Here's how the part is built. I have some questions about the finished solid (model axes, mm). Face numbers are marked on the shaded views. A direction names the side the tool comes from. Round coordinates to 2 decimals unless told otherwise and drop trailing zeros. Write each loop counter-clockwise with the first axis right and the second up, starting at its lowest first coordinate (ties: lowest second). Pieces come first, ordered by that corner, then holes. Notation, with made-up numbers: (7.5, 85.25) -> (34.5, 85.25) arc R8 ccw to (34.5, 94.25) -> close; hole circle Ø10 at (71.25, -36). An arc over 180 degrees is marked (long way). Answer in a Markdown table with one row per item.
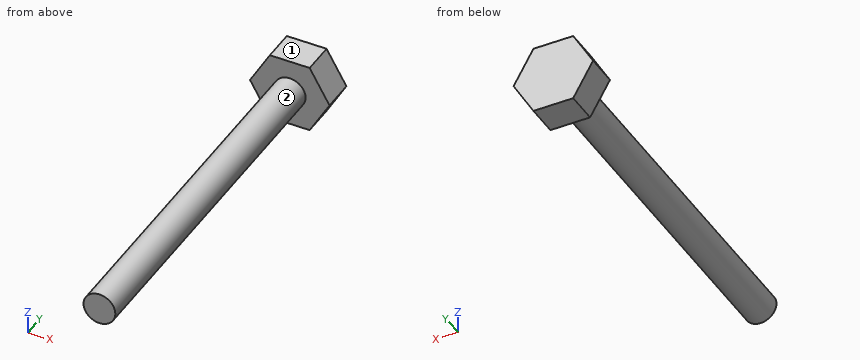
from build123d import *

# Parameters (mm, degrees)
SALIENTE_EXTRUIR1_DEPTH = 4
CROQUIS2_R              = 2
SALIENTE_EXTRUIR2_DEPTH = 45


with BuildPart() as part:
    # Croquis1 → Saliente-Extruir1 (new body)
    with BuildSketch(Plane(origin=(0, 0, 0), x_dir=(1, 0, 0), z_dir=(0, 1, 0))):
        Polygon((5, 0), (2.5, 4.330127019), (-2.5, 4.330127019), (-5, 0), (-2.5, -4.330127019), (2.5, -4.330127019), align=None)
    extrude(amount=SALIENTE_EXTRUIR1_DEPTH)

    # Croquis2 → Saliente-Extruir2 (add)
    with BuildSketch(Plane.XZ):
        Circle(CROQUIS2_R)
    extrude(amount=SALIENTE_EXTRUIR2_DEPTH)


solid = part.part
1) I want a section at A-A, the plane x = 0. List the corners of the cut face in (y, z) for me.
Response:
| item | result |
|---|---|
| outline | (-45, -2) -> (0, -2) -> (0, -4.33) -> (4, -4.33) -> (4, 4.33) -> (0, 4.33) -> (0, 2) -> (-45, 2) -> close |
2) For pin 1 (6 mm diameter, centred on x = 0, y = -30, fed in from -Z); pin 2 (1.5 mm diameter, centred on y = -32, z = -1, fed in from -X); pin 3 (2 mm diameter, centred on x = 2, y = -32, fed in from -Z), each with a flat end and sliding along its axis, tell me the tip position at first contact or that it passes through.
Response:
| item | result |
|---|---|
| pin 1 | stops at z = -2 |
| pin 2 | stops at x = -1.98 |
| pin 3 | stops at z = -1.73 |
3) Which directions (+Z, -Z, +X, -X, +Y, -Y) give clear straight access to the entire face, cutting with the end or side of a thin tool? Please do the marked faces 1 and 2.
Response:
| item | result |
|---|---|
| face 1 | +Z, +X, -X, +Y, -Y |
| face 2 | -Y |
4) I want a section at D-D, the plane x = 3.75. List the corners of the cut face in (y, z) for me.
Response:
| item | result |
|---|---|
| outline | (0, -2.17) -> (4, -2.17) -> (4, 2.17) -> (0, 2.17) -> close |
5) I want a section at C-C, the plane z = 3.75. List the corners of the cut face in (x, y) for me.
Response:
| item | result |
|---|---|
| outline | (-2.83, 0) -> (2.83, 0) -> (2.83, 4) -> (-2.83, 4) -> close |
6) I need wall thicknesses on line 1 (Y direction, x = -3.5, z = -1.75); line 2 (X direction, y = -27.5, z = -1); line 3 (Z direction, x = -1.25, y = -30). Which ranges of each line are inside material? Lowest first, please. Write a range as [from, to].
Response:
| item | result |
|---|---|
| line 1 | y = [0, 4] |
| line 2 | x = [-1.73, 1.73] |
| line 3 | z = [-1.56, 1.56] |
7) I want a section at B-B, the plane y = -35. List the corners of the cut face in (x, z) for me, and give its area (3 significant figures).
Response:
| item | result |
|---|---|
| outline | circle Ø4 at (0, 0) |
| area | 12.6 mm^2 |
